Here's how the part is built. I have some questions about the finished solid (model axes, mm). Coordinates: 2 decimals unless noted, no trailing zeros. Write each loop counter-clockwise with the first axis right and the second up, starting at its lowest first coordinate (ties: lowest second). Pieces come first, ordered by that corner, then holes.
(1) Imagine slicing it at A-A, the plane x = 8. List the corners of the cut face in (y, z) for me (3 decimals), plus the area to 3 significant figures.
(2) Please list where these lines run through material, in increasing order: probe 1 along Y at (x, z) = (4.5, 1) (3 decimals); probe 2 along X at (y, z) = (9.5, 2.6); probe 3 along Z at (x, y) = (36, 5).
(3) Imagine slicing it at C-C, the plane x = 27. List the corners of the cut face in (y, z) for me.
(4) For pin 1 Ø5 at (x, y) = (14.5, 9) entering from -Z; pin 2 Ø1.6 at (y, z) = (14.5, 1.5) entering from -X; pin 3 Ø5.5 at (x, y) = (13.5, 11) entering from +Z; pin 4 Ø2 at (x, z) = (29, 1) entering from -Y, each with a flat end and sliding along its axis, tell me the tip position at first contact or that it passes through.
(5) Imagine slicing it at B-B, the plane y = 5.25. List the corners of the cut face in (x, z) for me, plus the area to 3 significant figures.
Autodesk Inventor part; units mm, degrees
ref_plane "Work Plane2" through (0, 0, 3) normal (0, 0, 1) x (1, 0, 0)
ref_plane "YZ Plane" through (0, 0, 0) normal (1, 0, 0) x (0, 1, 0)
ref_plane "XZ Plane" through (0, 0, 0) normal (0, 1, 0) x (-1, 0, 0)
sketch "Sketch1" plane through (0, 0, 0) normal (0, 0, 1) x (1, 0, 0)
  line L0 (0, 0) -> (43, 0)
  line L1 (43, 0) -> (43, 19)
  line L2 (43, 19) -> (0, 19)
  line L3 (0, 19) -> (0, 0)
  dimension "d0" = 43
extrude "Extrusion1" add sketch "Sketch1" along normal blind 2
fillet "Fillet1" radius 2 4 edges at (43, 19, 1) (43, 0, 1) (0, 19, 1) (0, 0, 1)
sketch "Sketch3" plane through (0, 2, 0) normal (-1, 0, 0) x (0, 0, 1)
  line L0 (2, 0) -> (0, 0) construction
  line L1 (2, 15) -> (2, 0) construction
  line L2 (0, 0) -> (2, 15) construction
  line L3 (0, 15) -> (2, 0) construction
  circle A0 centre (1, 7.5) radius 2
  point P0 (0, -2)
  dimension "d4" = 4
extrude "Extrusion2" add sketch "Sketch3" along normal blind 2 and the other way blind 10
sketch "Sketch4" plane through (-2, 9.5, 1) normal (-1, 0, 0) x (0, 0, 1)
  point P0 (-1, -9.5)
  point P1 (0, 0)
hole "Hole1" at (-2, 9.5, 1) direction (1, 0, 0) diameter 2.85 depth 10.4 tip angle 118
ref_plane "Work Plane2" through (0, 0, 3) normal (0, 0, 1) x (1, 0, 0)
ref_plane "Work Plane1" through (0, 0, 1) normal (0, 0, 1) x (1, 0, 0)
sketch "Sketch6" plane through (0, 0, 3) normal (0, 0, 1) x (1, 0, 0)
  line L0 (-2, 11.5) -> (-2, 7.5) construction
  line L1 (0, 7.5) -> (0, 7.7679) construction
  line L2 (-2, 11.5) -> (0, 7.5) construction
  line L3 (0, 7.5) -> (-2, 7.5) construction
  line L4 (-2, 7.5) -> (0, 11.5) construction
  line L5 (0, 11.5) -> (-2, 11.5) construction
  point P0 (0, 0)
  point P1 (-1, 9.5)
hole "Hole2" at (-1, 9.5, 3) direction (0, 0, -1) diameter 0.5 depth 3.5 tip angle 118
properties part number "UntererRührer"
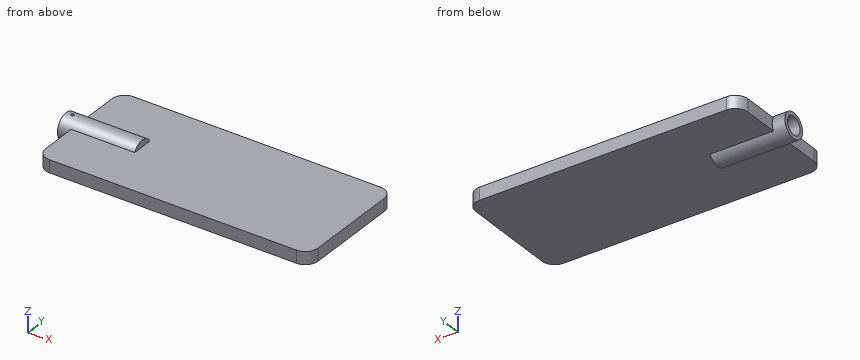
Recorded:
1. outline: (0, 0) - (7.768, 0) arc R2 ccw to (11.232, 0) - (19, 0) - (19, 2) - (11.232, 2) arc R2 ccw to (7.768, 2) - (0, 2) - close; hole circle Ø2.85 at (9.5, 1)
1. area: 36.5 mm2
2. probe 1: y = 0 to 8.075, 10.925 to 19
2. probe 2: x = -2 to -1.25, -0.75 to 10
2. probe 3: z = 0 to 2
3. outline: (0, 0) - (19, 0) - (19, 2) - (0, 2) - close
4. pin 1: stops at z = 0
4. pin 2: stops at x = 0
4. pin 3: stops at z = 2
4. pin 4: stops at y = 0
5. outline: (0, 0) - (43, 0) - (43, 2) - (0, 2) - close
5. area: 86.0 mm2
